Verification items for the finished model (mm, model axes). Face numbers are marked on the shaded views. A direction names the side the tool comes from. Give positions to 0.01 mm unless a question says otherwise; leave off trailing zeros. Order: outer loops, then holes, each group sorted by start corner. A loop starts at its lowest first (then second) coordinate and runs counter-clockwise, first axis right, second up. Notation, with made-up numbers: (59.25, 41) -> (115.25, 41) arc R9 cw to (115.25, 53) -> close; hole circle Ø11 at (7, 25). An arc over 180 degrees is marked (long way). One line per question, with ' | ' between items. Start each with the question number.
Q1. Section check D-D on y = 5. Record the cut outline in (x, z).
Q2. Material ranges on probe 1 along X at (y, z) = (48, -19); probe 2 along Y at (x, z) = (-63, -107.5), recorded low to high. Write a range as [from, to].
Q3. Section check C-C on x = -52. Record the cut outline in (y, z).
Q4. Section check B-B on z = 22. Record the cut outline in (x, y).
Q5. Access from +Z, -Z, +X, -X, +Y, -Y to the whole of each face (thin tool, end or side, straight path). Record for the marked faces 1, 2, 3, 4 and 5.
Q6. Mould release check, pull along Z, two halves, no side actions. Record for the marked faces 6, 7 and 8: released by +Z, released by -Z, zero draft, split by the parting line, or undercut.
Q7. Go/stop test with flat-tipped pins: pin 1 (10 mm diameter, centred on y = 60.5, z = -121, fed in from +X); pin 2 (6 mm diameter, centred on y = 6.5, z = -46.5, fed in from -X); pin 3 (2.5 mm diameter, centred on x = -93, y = 58, fed in from +Z). Record where each tip stops, or that it passes through.
Q8. Section check A-A on x = -100. Record the cut outline in (y, z).
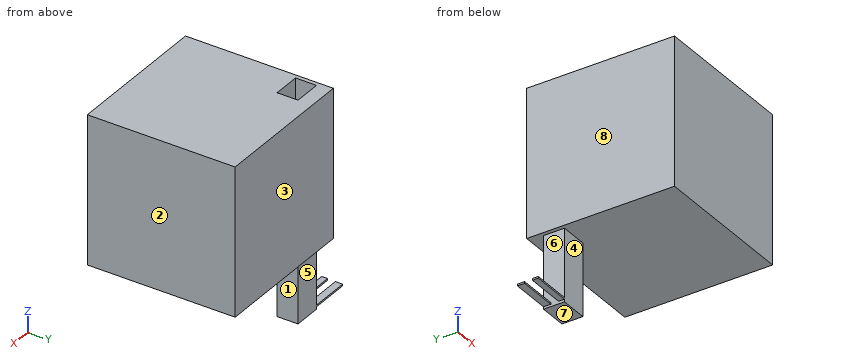
from build123d import *

# Parameters (mm, degrees)
F1_W       = 152.4
F1_H       = 152.4
F2_DEPTH   = 76.2
F3_W       = 28.6219716072
F3_H       = 21.6014906764
F2_FACE1_W = 152.4
F2_FACE1_H = 152.4
F4_DEPTH   = 81.28
F5_W       = 28.6219716072
F5_H       = 21.6014906764
F6_DEPTH   = 74.676
F7_W       = 7.5074806809
F7_H       = 1.7182230949
F7_W_2     = 6.0756318271
F7_H_2     = 1.7272
F8_DEPTH   = 40.64


# Not quite as in the source:
# - a variable given as a bare number and used for a length is read in inches; the dataset says mm whatever the document's units were


with BuildPart() as f2:
    # F1 (on Front) → F2 (new body, symmetric)
    with BuildSketch(Plane.XZ):
        Rectangle(F1_W, F1_H)
    extrude(amount=F2_DEPTH, both=True)

    # F3 (on face) + F2_face1 (on face) → F4 (cut)
    with BuildSketch(Plane.XY.offset(76.2)):
        with Locations((-57.7839799225, 50.7634989917)):
            Rectangle(F3_W, F3_H)
    with BuildSketch(Plane(origin=(0, 0, -76.2), x_dir=(1, 0, 0), z_dir=(0, 0, -1))):
        Rectangle(F2_FACE1_W, F2_FACE1_H)
    extrude(amount=-F4_DEPTH, dir=(0, 0, 1), mode=Mode.SUBTRACT)

    # F5 (on face) → F6 (join)
    with BuildSketch(Plane(origin=(0, 0, -76.2), x_dir=(1, 0, 0), z_dir=(0, 0, -1))):
        with Locations((-57.7839799225, -50.7634989917)):
            Rectangle(F5_W, F5_H)
    extrude(amount=F6_DEPTH)

    # F7 (on face) → F8 (join)
    with BuildSketch(Plane(origin=(-72.0949657261, 0, 0), x_dir=(0, -1, 0), z_dir=(-1, 0, 0))):
        with Locations((-57.8105039895, -147.6161032915)):
            Rectangle(F7_W, F7_H)
        with Locations((-43.0005695671, -147.3252443232)):
            Rectangle(F7_W_2, F7_H_2)
    extrude(amount=F8_DEPTH)


solid = f2.part
Filled in:
1) outline: (-76.2, -76.2) -> (76.2, -76.2) -> (76.2, 76.2) -> (-76.2, 76.2) -> close
2) probe 1: [-76.2, 76.2] | probe 2: [39.96, 61.56]
3) outline: (-76.2, -76.2) -> (39.96, -76.2) -> (39.96, -150.88) -> (61.56, -150.88) -> (61.56, -76.2) -> (76.2, -76.2) -> (76.2, 76.2) -> (61.56, 76.2) -> (61.56, -5.08) -> (39.96, -5.08) -> (39.96, 76.2) -> (-76.2, 76.2) -> close
4) outline: (-76.2, -76.2) -> (76.2, -76.2) -> (76.2, 76.2) -> (-76.2, 76.2) -> close; hole (-72.09, 39.96) -> (-43.47, 39.96) -> (-43.47, 61.56) -> (-72.09, 61.56) -> close
5) face 1: -Z, +X, +Y, -Y | face 2: +Z, -Z, +X, +Y, -Y | face 3: +Z, -Z, +X, -X, +Y | face 4: -Z, +X, -X, -Y | face 5: -Z, +X, -X, +Y
6) face 6: undercut | face 7: released by -Z | face 8: zero draft
7) pin 1: x = -43.47 | pin 2: x = -76.2 | pin 3: z = -146.76
8) outline: (39.96, -148.19) -> (46.04, -148.19) -> (46.04, -146.46) -> (39.96, -146.46) -> close; (54.06, -148.48) -> (61.56, -148.48) -> (61.56, -146.76) -> (54.06, -146.76) -> close
